Work out the finished part from the listing and answer in its coordinate system (mm). A direction names the side the tool comes from. Coordinates: 2 decimals unless noted, no trailing zeros. Write each loop counter-clockwise with the first axis right and the second up, starting at its lowest first coordinate (ties: lowest second). Pieces come first, ordered by that corner, then holes. Notation, with made-up numbers: M -39,60.25 L 15,60.25 A6 cw 15,66.25 Z; hole C -6,49 d5. An arc over 180 degrees is marked long. Use CSV: the item, a comma, the result in double quotes.
from build123d import *

# Parameters (mm, degrees)
SKETCH_1_R               = 5
EXTRUDE_1_DEPTH          = 7.5
SKETCH_1_5_R             = 2.75
CUT_EXTRUDE_1_DEPTH      = 6.5
SKETCH_1_6_R             = 0.5
CUT_EXTRUDE_2_DEPTH      = 11.307764064
SKETCH_1_7_R             = 0.35
CUT_EXTRUDE_3_DEPTH      = 2
PATTERN_CIRCULAR_1_COUNT = 4


with BuildPart() as part:
    # Sketch 1 → Extrude 1 (new body)
    with BuildSketch(Plane(origin=(0, 0, 0), x_dir=(1, 0, 0), z_dir=(0, 1, 0))):
        with Locations(Location((0, 0, 0), (0, 0, 270))):
            Circle(SKETCH_1_R)
    extrude(amount=EXTRUDE_1_DEPTH)

    # Sketch 1_5 → Cut-Extrude 1 (cut)
    with BuildSketch(Plane(origin=(0, 0, 0), x_dir=(1, 0, 0), z_dir=(0, 1, 0))):
        with Locations(Location((0, 0, 0), (0, 0, 90))):
            Circle(SKETCH_1_5_R)
    extrude(amount=CUT_EXTRUDE_1_DEPTH, mode=Mode.SUBTRACT)

    # Sketch 1_6 → Cut-Extrude 2 (cut, through all)
    with BuildSketch(Plane(origin=(0, 0, 0), x_dir=(1, 0, 0), z_dir=(0, 1, 0))):
        with Locations(Location((0, 0, 0), (0, 0, 270))):
            Circle(SKETCH_1_6_R)
    extrude(amount=CUT_EXTRUDE_2_DEPTH, mode=Mode.SUBTRACT)

    # Sketch 1_7 → Cut-Extrude 3 (cut)
    with BuildSketch(Plane(origin=(0, 0, 0), x_dir=(1, 0, 0), z_dir=(0, 1, 0))):
        with Locations(Location((-3.875, 0, 0), (0, 0, 270))):
            Circle(SKETCH_1_7_R)
    cut_extrude_3 = extrude(amount=CUT_EXTRUDE_3_DEPTH, mode=Mode.SUBTRACT)

    # Pattern Circular 1: Cut-Extrude 3 ×4 about axis
    pattern_circular_1_axis = Axis((0, 0, 0), (0, 1, 0))
    for i in range(1, PATTERN_CIRCULAR_1_COUNT):
        add(cut_extrude_3.rotate(pattern_circular_1_axis, i * 360 / PATTERN_CIRCULAR_1_COUNT), mode=Mode.SUBTRACT)


solid = part.part
Item 1: Given pin 1 (1 mm diameter, centred on x = 2, z = -0.5, fed in from -Y); pin 2 (2 mm diameter, centred on y = 3, z = -2, fed in from +X), each flat-ended and moving along its own axis, determine where each tip first touches the part or whether it passes through.
Answer:
pin 1,"stops at y = 6.5"
pin 2,"stops at x = 4.9"
Item 2: For a pull along Z with two mould halves and no side action, classify faces 3 (the face through (0, 7.5, 1)), 4 (the face through (-0.488, 6.993, -0.108)), 5 (the face through (-4.88, 3.7, -1.08)) as released by +Z, released by -Z, zero draft, split by the parting line, or undercut.
Answer:
face 3,"zero draft"
face 4,"undercut"
face 5,"split by the parting line"
Item 3: The part is cut by section B-B (z = 0). Write down the section's boundary in (x, y) (3 decimals), then the cut area to 4 significant figures.
Answer:
outline,"M -5,0 L -4.225,0 L -4.225,2 L -3.525,2 L -3.525,0 L -2.75,0 L -2.75,6.5 L -0.5,6.5 L -0.5,7.5 L -5,7.5 Z; M 0.5,6.5 L 2.75,6.5 L 2.75,0 L 3.525,0 L 3.525,2 L 4.225,2 L 4.225,0 L 5,0 L 5,7.5 L 0.5,7.5 Z"
area,"35.45 mm2"
Item 4: The part is cut by section A-A (x = 0). Write down the section's boundary in (y, z) (3 decimals).
Answer:
outline,"M 0,-5 L 7.5,-5 L 7.5,-0.5 L 6.5,-0.5 L 6.5,-2.75 L 0,-2.75 L 0,-3.525 L 2,-3.525 L 2,-4.225 L 0,-4.225 Z; M 0,2.75 L 6.5,2.75 L 6.5,0.5 L 7.5,0.5 L 7.5,5 L 0,5 L 0,4.225 L 2,4.225 L 2,3.525 L 0,3.525 Z"
Item 5: The part is cut by section C-C (y = 2.5). Write down the section's boundary in (x, z), then the cut area to 3 significant figures.
Answer:
outline,"C 0,0 d10; hole C 0,0 d5.5"
area,"54.8 mm2"
Item 6: A tool of negligible diameter and unlimited length cuts with its end or side. For faces 1 (the face through (-2.2, 0, 2.2)), 2 (the face through (1, 6.5, 0)), from which of +Z, -Z, +X, -X, +Y, -Y can it reach the whole face along a straight path? Write none if from no direction.
Answer:
face 1,"+Z, -Z, +X, -X, -Y"
face 2,"-Y"
Item 7: The part is cut by section D-D (x = 1.25). Write down the section's boundary in (y, z), then the cut area to 3 significant figures.
Answer:
outline,"M 0,-4.84 L 7.5,-4.84 L 7.5,4.84 L 0,4.84 L 0,2.45 L 6.5,2.45 L 6.5,-2.45 L 0,-2.45 Z"
area,"40.8 mm2"
Item 8: Consider probe 1 along X at (y, z) = (1.6, 0) (3 decimals); probe 2 along X at (y, z) = (7, 0); probe 3 along Y at (x, z) = (-1.5, -2). Determine where each line is inside the solid, lowest interval first.
Answer:
probe 1,"x = -5 to -4.225, -3.525 to -2.75, 2.75 to 3.525, 4.225 to 5"
probe 2,"x = -5 to -0.5, 0.5 to 5"
probe 3,"y = 6.5 to 7.5"
